Design review of the part built by this model. Coordinates are the model's own, in mm. A direction names the side the tool comes from. Round coordinates to 2 decimals unless told otherwise and drop trailing zeros. Write each loop counter-clockwise with the first axis right and the second up, starting at its lowest first coordinate (ties: lowest second). Pieces come first, ordered by that corner, then holes. Notation, with made-up numbers: (2.25, 25) -> (32.25, 25) arc R27 ccw to (32.25, 46) -> close; hole circle Ø11 at (80, 32.25). An arc over 180 degrees is marked (long way). Write item = value, one per line. Start each with the question number.
Item 1: For pin 1 Ø5.5 at (y, z) = (8.5, 164) entering from -X; pin 2 Ø8 at (y, z) = (19.5, 270) entering from -X; pin 3 Ø14.5 at (x, z) = (19, 246) entering from +Y; pin 4 Ø10 at (x, z) = (-1.5, 137.5) entering from +Y, all flat-tipped, find the tip position at first contact; note any pin that passes through.
Item 2: Add section C-C, the plane y = 27. State the section outline as (x, z) points, then the cut area to 3 significant figures.
Item 3: Mouldability with a two-part tool opening along Y and no side actions: class faces 5 (the flat face through (-16, 5, 197)), 6 (the cylindrical face through (-0.351, 36.293, 197.2)), 7 (the flat face through (0, 14, 0)) as released by +Y, released by -Y, zero draft, split by the parting line, or undercut.
Item 4: Add section A-A, the plane z = 83. State the section outline as (x, y) points, then the cut area to 3 significant figures.
Item 5: Add section B-B, the plane x = 15.5. State the section outline as (y, z) points.
Item 6: Machinability: for faces 1 (the flat face through (16, 5, 197)), 2 (the flat face through (6.45, 14.36, 197.2)), 3 (the flat face through (0, 0, 197)), 4 (the flat face through (-6.45, 14.36, 197.2)), which of the approach directions +Z, -Z, +X, -X, +Y, -Y give a long, thin tool a straight path to every point of the face, cutting with its end or side? Answer none if there is none.
Item 7: To check wall thickness, follow L1, parallel to Y at x = -16, z = 244; L2, parallel to Y at x = -1, z = 200; L3, parallel to X at y = 26, z = 193. State the ranges of each line that lie inside material, in increasing order.
Autodesk Inventor part; units mm, degrees
ref_plane "YZ Plane" through (0, 0, 0) normal (1, 0, 0) x (0, 1, 0)
ref_plane "XZ Plane" through (0, 0, 0) normal (0, 1, 0) x (-1, 0, 0)
ref_plane "XY Plane" through (0, 0, 0) normal (0, 0, 1) x (1, 0, 0)
sketch "Sketch1" plane through (0, 0, 0) normal (0, 0, 1) x (1, 0, 0)
  line L0 (-22.5, 0) -> (22.5, 0)
  line L1 (22.5, 0) -> (22.5, 5)
  line L2 (-22.5, 0) -> (-22.5, 5)
  line L3 (-22.5, 5) -> (-9.5, 5)
  line L4 (22.5, 5) -> (9.5, 5)
  line L5 (-9.5, 5) -> (-9.5, 10)
  line L6 (9.5, 5) -> (9.5, 10)
  arc A0 (4, 18.6042) -> (-4, 18.6042) centre (0, 27) ccw
  line L7 (4, 18.6042) -> (8.9676, 10)
  line L8 (-4, 18.6042) -> (-8.9676, 10)
  line L9 (-9.5, 10) -> (9.5, 10) construction
  line L10 (-8.9676, 10) -> (-9.5, 10) construction
  line L11 (-8.9676, 10) -> (-9.5, 10)
  line L12 (8.9676, 10) -> (9.5, 10)
  line L13 (-11.4601, 5) -> (-11.4601, 0) construction
  line L14 (-16.9601, 5) -> (-16.9601, 0) construction
  line L15 (13.0399, 5) -> (13.0399, 0) construction
  line L16 (18.5399, 5) -> (18.5399, 0) construction
  arc A1 (-4, 18.6042) -> (4, 18.6042) centre (0, 27) ccw construction
  point P0 (0, 0)
  point P1 (0, 0)
  point P2 (0, 17.7)
  point P3 (15.7899, 5)
  point P4 (-14.2101, 5)
  dimension "B" = 45
  dimension "t" = 5
  dimension "d2" = 5
  dimension "dimensionf" = 19
  dimension "d4" = 13
  dimension "Y" = 10
  dimension "d6" = 5
  dimension "d" = 18.6
  dimension "e" = 22.5
  dimension "dimensionH" = 17.7
  dimension "dimensionh" = 27
  dimension "x" = 8
  dimension "d16" = 4
  dimension "dimensionc" = 30
  dimension "d21" = 6.7101
  dimension "s1" = 5.5
  dimension "d23" = 5.5
  dimension "d24" = 2.75
  dimension "d25" = 2.75
extrude "Extrusion1" add sketch "Sketch1" along normal blind 400
equation "\"d2\" = t"
properties part number "sbr20_400mm"
Result set:
q1.pin_1 = -9.5
q1.pin_2 = -8.62
q1.pin_3 = 5
q1.pin_4 = 36.3
q2.outline = (-9.3, 0) -> (9.3, 0) -> (9.3, 400) -> (-9.3, 400) -> close
q2.area = 7,440 mm²
q3.face_5 = released by +Y
q3.face_6 = undercut
q3.face_7 = zero draft
q4.outline = (-22.5, 0) -> (22.5, 0) -> (22.5, 5) -> (9.5, 5) -> (9.5, 10) -> (8.97, 10) -> (4, 18.6) arc R9.3 ccw (long way) to (-4, 18.6) -> (-8.97, 10) -> (-9.5, 10) -> (-9.5, 5) -> (-22.5, 5) -> close
q4.area = 698 mm²
q5.outline = (0, 0) -> (5, 0) -> (5, 400) -> (0, 400) -> close
q6.face_1 = +Z, -Z, +X, +Y
q6.face_2 = +Z, -Z, +X
q6.face_3 = +Z, -Z, +X, -X, -Y
q6.face_4 = +Z, -Z, -X
q7.L1 = 0 to 5
q7.L2 = 0 to 36.25
q7.L3 = -9.25 to 9.25
